Design review of the part built by this model. Coordinates are the model's own, in mm. Face numbers are marked on the shaded views. A direction names the side the tool comes from. Coordinates: 2 decimals unless noted, no trailing zeros. Write each loop counter-clockwise with the first axis right and the second up, starting at its lowest first coordinate (ties: lowest second). Pieces come first, ordered by that corner, then holes. Notation, with made-up numbers: (-10.75, 78) -> (9.25, 78) arc R23 cw to (9.25, 106) -> close; hole circle Ø10 at (36.25, 27). An arc over 180 degrees is marked (long way). Write item = value, one per line. Start each with the question number.
```python
from build123d import *

# Parameters (mm, degrees)
ZAOKR_GLENIE1_R            = 2
WYTNIJ_WYCI_GNI_CIE1_DEPTH = 134


with BuildPart() as part:
    # Szkic2 → Obrót1 (revolve)
    with BuildSketch(Plane.XY):
        Polygon((0, 0), (0, 25), (19, 25), (19, 40), (47.5, 40), (50, 37.5), (83, 37.5), (85.5, 40), (114, 40), (114, 25), (133, 25), (133, 0), align=None)
    revolve(axis=Axis((133, 0, 0), (-1, 0, 0)))

    # Zaokrąglenie1
    zaokr_glenie1_edges = [part.edges().sort_by_distance(p)[0] for p in [
        (114, -25, 0),
        (19, -25, 0),
    ]]
    fillet(zaokr_glenie1_edges, radius=ZAOKR_GLENIE1_R)

    # Szkic3 → Wytnij-wyciągnięcie1 (cut, through all)
    with BuildSketch(Plane.ZY):
        with BuildLine():
            Line((0, 0), (0, 7))
            Line((0, 7), (-12, 7))
            ThreePointArc((-12, 7), (-15, 10), (-12, 13))
            Line((-12, 13), (0, 13))
            Line((0, 13), (0, 40))
            ThreePointArc((0, 40), (28.284271247, 28.284271247), (40, 0))
            Line((40, 0), (0, 0))
        make_face()
    extrude(amount=-WYTNIJ_WYCI_GNI_CIE1_DEPTH, mode=Mode.SUBTRACT)


solid = part.part
```
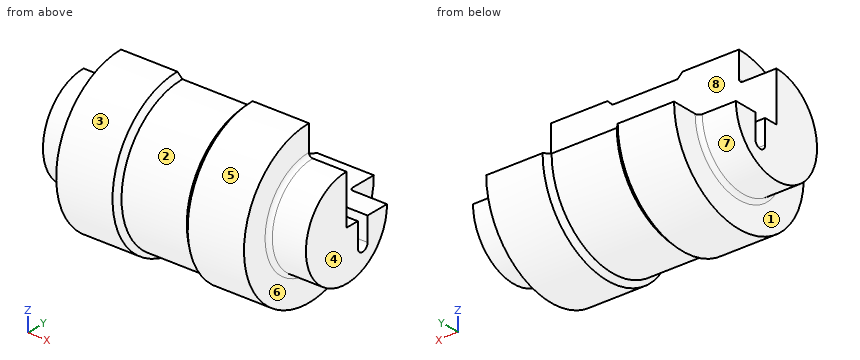
(1) Mouldability with a two-part tool opening along X and no side actions: class the marked faces 1, 2 and 3 as pulls with the +X half, pulls with the -X half, needs draft (parallel to the pull), parting line crosses it, or undercut.
(2) For pin 1 Ø3 at (x, y) = (71, 31) entering from -Z; pin 2 Ø3 at (y, z) = (-15.5, -27.5) entering from -X; pin 3 Ø9.5 at (x, z) = (33.5, -8.5) entering from -Y, all flat-tipped, find the tip position at first contact; note any pin that passes through.
(3) For line 1 (X direction, y = -19, z = -33.5); line 2 (Z direction, x = 101, y = 1.5); line 3 (Y direction, x = 11, z = -12.5), list the stretches that pass through material, from the lowest coordinate up.
(4) Take a section at B-B, the plane x = 36. State the section outline as (y, z) points.
(5) Take a section at A-A, the plane x = 58. State the section outline as (y, z) points, then the cut area to 3 significant figures.
(6) For the marked faces 4, 5, 6, 7 and 8, list the 3-axis set-ups (+Z, -Z, +X, -X, +Y, -Y) from which the entire face can be reached by the end or side of a thin tool; tool diameter is ignored.
Report:
q1.face_1 = pulls with the -X half
q1.face_2 = undercut
q1.face_3 = needs draft
q2.pin_1 = -23.15
q2.pin_2 = 19
q2.pin_3 = -39.82
q3.line_1 = 19 to 48.99, 84.01 to 114
q3.line_2 = -39.97 to 0
q3.line_3 = -21.65 to 7.04, 12.96 to 21.65
q4.outline = (0, 0) -> (0, 40) arc R40 ccw (long way) to (40, 0) -> (13, 0) -> (13, -12) arc R3 cw to (7, -12) -> (7, 0) -> close
q5.outline = (0, 0) -> (0, 37.5) arc R37.5 ccw (long way) to (37.5, 0) -> (13, 0) -> (13, -12) arc R3 cw to (7, -12) -> (7, 0) -> close
q5.area = 3,230 mm2
q6.face_4 = +Z, -Z, +X, +Y, -Y
q6.face_5 = +X, -X
q6.face_6 = +X
q6.face_7 = -X
q6.face_8 = +Z, +X, -X, +Y
